Build history of the part. All positions in model axes, mm. A direction names the side the tool comes from. Round coordinates to 2 decimals unless told otherwise and drop trailing zeros. Write each loop counter-clockwise with the first axis right and the second up, starting at its lowest first coordinate (ties: lowest second). Pieces come first, ordered by that corner, then holes. Notation, with made-up numbers: M -4,62 L 52,62 A16 cw 52,70 Z; hole C 82,23.5 d1. An arc over 180 degrees is marked long. Write item = value, one per line. Start each with the question number.
Q1. Probe L1, parallel to X at y = 0, z = -3.25; L2, parallel to X at y = 0, z = 2.25; L3, parallel to X at y = 9.5, z = 0.5. List the from-to ranges inside material, lowest first.
Q2. Band-saw the part on B-B on x = -10.5. Write the cut outline in (y, z).
Q3. Band-saw the part on D-D on y = -10.5. Write the cut outline in (x, z), plus the area to 3 significant figures.
Q4. Tool access for faces 5 (the cylindrical face through (7.865, 12.592, 0.07)), 6 (the cylindrical face through (-2.44, 0.05, -0.54)), 7 (the flat face through (-8.52, 14.76, -0.07)): list every direction of +Z, -Z, +X, -X, +Y, -Y with a clear straight run to the whole face (end or side of a thin tool).
Q5. Drop flat-ended pins along their axis: P1, Ø1.5, axis at x = -4.5, z = 2, coming from the +Y side; P2, Ø1, axis at x = 3.5, z = 4, coming from the -Y side; P3, Ø4, axis at x = 11.5, z = 3.5, coming from the +Y side. Give the stop position or say it passes through.
Q6. Band-saw the part on C-C on z = 3.25. Write the cut outline in (x, y).
Q7. Band-saw the part on A-A on y = 0. Write the cut outline in (x, z).
Q8. Pull direction X, two halves, no side cores. Call faces 1 (the flat face through (9.392, 13.867, -0.07)), 2 (the cylindrical face through (-0.5, -14.29, 3.26)), 3 (the flat face through (0, 16, 0)), 4 (the flat face through (-9.374, 13.837, -0.07)): released by +X, released by -X, zero draft, split by the parting line, or undercut.
```python
from build123d import *

# Parameters (mm, degrees)
BOSS_EXTRUDE1_DEPTH             = 5
BOSS_EXTRUDE1_DEPTH_BACK        = 5
SKETCH2_R                       = 2.5
BOSS_EXTRUDE2_DEPTH             = 16
BOSS_EXTRUDE2_DIRECTION_2_REACH = 24.483
FILLET2_R                       = 2
FILLET3_R                       = 2


with BuildPart() as part:
    # Sketch1 → Boss-Extrude1 (new, two sides: drawn at the far end of the back side and taken through both)
    with BuildSketch(Plane.XY.offset(-BOSS_EXTRUDE1_DEPTH_BACK)):
        with BuildLine():
            Line((7.15, 12.384163274), (8.942753286, 15.489303051))
            ThreePointArc((8.942753286, 15.489303051), (9.47564549, 15.212840275), (10, 14.920508076))
            Line((10, 14.920508076), (8.765969771, 12.783105021))
            ThreePointArc((8.765969771, 12.783105021), (0, -15.5), (-8.765969771, 12.783105021))
            Line((-8.765969771, 12.783105021), (-10, 14.920508076))
            ThreePointArc((-10, 14.920508076), (-9.47564549, 15.212840275), (-8.942753286, 15.489303051))
            Line((-8.942753286, 15.489303051), (-7.15, 12.384163274))
            ThreePointArc((-7.15, 12.384163274), (0, -14.3), (7.15, 12.384163274))
        make_face()
    extrude(amount=BOSS_EXTRUDE1_DEPTH + BOSS_EXTRUDE1_DEPTH_BACK)

    # Sketch2 → Boss-Extrude2 (add)
    with BuildSketch(Plane(origin=(0, 0, 0), x_dir=(1, 0, 0), z_dir=(0, 1, 0))):
        with Locations(Location((0, 0, 0), (0, 0, 270))):
            Circle(SKETCH2_R)
    extrude(amount=BOSS_EXTRUDE2_DEPTH)

    # Sketch2 → Boss-Extrude2 direction 2 (add, up to next)
    with BuildSketch(Plane(origin=(0, 0, 0), x_dir=(1, 0, 0), z_dir=(0, 1, 0)), mode=Mode.PRIVATE) as boss_extrude2_direction_2_sk1:
        with Locations(Location((0, 0, 0), (0, 0, 270))):
            Circle(SKETCH2_R)
    boss_extrude2_direction_2_tool1 = extrude(boss_extrude2_direction_2_sk1.sketch, amount=-BOSS_EXTRUDE2_DIRECTION_2_REACH, mode=Mode.PRIVATE) - part.part
    add(boss_extrude2_direction_2_tool1.solids().sort_by_distance((0, 0, 0))[0])

    # Fillet2
    fillet2_edges = [part.edges().sort_by_distance(p)[0] for p in [
        (0, 16, -2.5),
    ]]
    fillet(fillet2_edges, radius=FILLET2_R)

    # Fillet3
    fillet3_edges = [part.edges().sort_by_distance(p)[0] for p in [
        (-7.15, 12.384163274, 0),
        (7.15, 12.384163274, 0),
    ]]
    fillet(fillet3_edges, radius=FILLET3_R)


solid = part.part
```
Conclusion:
q1.L1 = -15.5 to -14.3, 14.3 to 15.5
q1.L2 = -15.5 to -14.3, -1.09 to 1.09, 14.3 to 15.5
q1.L3 = -12.25 to -10.69, -2.45 to 2.45, 10.69 to 12.25
q2.outline = M -11.4,-5 L -9.71,-5 L -9.71,5 L -11.4,5 Z; M 9.71,-5 L 11.4,-5 L 11.4,5 L 9.71,5 Z
q3.outline = M -11.4,-5 L -9.71,-5 L -9.71,5 L -11.4,5 Z; C 0,0 d5; M 9.71,-5 L 11.4,-5 L 11.4,5 L 9.71,5 Z
q3.area = 53.5 mm^2
q4.face_5 = +Z, -Z
q4.face_6 = +Y
q4.face_7 = +Z, -Z, +Y
q5.P1 = -13.3
q5.P2 = -15.21
q5.P3 = 15.2
q6.outline = M -10,14.92 L -8.77,12.78 A15.5 ccw long 8.77,12.78 L 10,14.92 A20 ccw 8.94,15.49 L 8.09,14.01 A2 ccw 8.62,11.41 A14.3 cw long -8.62,11.41 A2 ccw -8.09,14.01 L -8.94,15.49 A20 ccw Z
q7.outline = M -15.5,-5 L -14.3,-5 L -14.3,5 L -15.5,5 Z; C 0,0 d5; M 14.3,-5 L 15.5,-5 L 15.5,5 L 14.3,5 Z
q8.face_1 = released by +X
q8.face_2 = undercut
q8.face_3 = zero draft
q8.face_4 = released by -X
